Geometry check sheet. Reference: the model listing, model coordinates, mm. Round coordinates to 2 decimals unless told otherwise and drop trailing zeros. Loops run counter-clockwise (first coordinate to the right, second up) from the corner with the lowest first, then second, coordinate; pieces in that order, holes last.
```python
from build123d import *

# Parameters (mm, degrees)
SKETCH1_W                 = 3
SKETCH1_H                 = 3
PLATE_THICKNESS_3MM_DEPTH = 3
SKETCH_1_W                = 10
SKETCH_1_H                = 3
SKETCH_1_W_2              = 3
SKETCH_1_H_2              = 5
CUT_EXTRUDE_1_DEPTH       = 3


with BuildPart() as part:
    # Sketch1 → Plate_thickness_3mm (new body)
    with BuildSketch(Plane.XY):
        Polygon((30, -55), (-30, -55), (-30, -58), (-43, -58), (-43, -55), (-41.5, -55), (-41.5, -50), (-43, -50), (-43, -46), (-47, -46), (-47, -50), (-48.5, -50), (-48.5, -55), (-47, -55), (-47, -58), (-60, -58), (-60, -55), (-90, -55), (-90, 55), (-60, 55), (-60, 58), (-47, 58), (-47, 55), (-48.5, 55), (-48.5, 50), (-47, 50), (-47, 46), (-43, 46), (-43, 50), (-41.5, 50), (-41.5, 55), (-43, 55), (-43, 58), (-30, 58), (-30, 55), (30, 55), (30, 58), (43, 58), (43, 55), (41.5, 55), (41.5, 50), (43, 50), (43, 46), (47, 46), (47, 50), (48.5, 50), (48.5, 55), (47, 55), (47, 58), (60, 58), (60, 55), (90, 55), (90, -55), (60, -55), (60, -58), (47, -58), (47, -55), (48.5, -55), (48.5, -50), (47, -50), (47, -46), (43, -46), (43, -50), (41.5, -50), (41.5, -55), (43, -55), (43, -58), (30, -58), align=None)
        with Locations((-60, -10.785)):
            Rectangle(SKETCH1_W, SKETCH1_H, mode=Mode.SUBTRACT)
        with Locations((60, -10.785)):
            Rectangle(SKETCH1_W, SKETCH1_H, mode=Mode.SUBTRACT)
        with Locations((-70.785, 0)):
            Rectangle(SKETCH1_W, SKETCH1_H, mode=Mode.SUBTRACT)
        with Locations((-49.215, 0)):
            Rectangle(SKETCH1_W, SKETCH1_H, mode=Mode.SUBTRACT)
        with Locations((-60, 10.785)):
            Rectangle(SKETCH1_W, SKETCH1_H, mode=Mode.SUBTRACT)
        with Locations((49.215, 0)):
            Rectangle(SKETCH1_W, SKETCH1_H, mode=Mode.SUBTRACT)
        with Locations((70.785, 0)):
            Rectangle(SKETCH1_W, SKETCH1_H, mode=Mode.SUBTRACT)
        with Locations((60, 10.785)):
            Rectangle(SKETCH1_W, SKETCH1_H, mode=Mode.SUBTRACT)
    extrude(amount=PLATE_THICKNESS_3MM_DEPTH)

    # 草图1 → 切除-拉伸1 (cut)
    with BuildSketch(Plane.XY.offset(3)):
        with Locations((-60, -10.785)):
            Rectangle(SKETCH_1_W, SKETCH_1_H)
        with Locations((-70.785, -2.5)):
            Rectangle(SKETCH_1_W_2, SKETCH_1_H_2)
        with Locations((-70.785, 2.5)):
            Rectangle(SKETCH_1_W_2, SKETCH_1_H_2)
        with Locations((-49.215, 2.5)):
            Rectangle(SKETCH_1_W_2, SKETCH_1_H_2)
        with Locations((-49.215, -2.5)):
            Rectangle(SKETCH_1_W_2, SKETCH_1_H_2)
        with Locations((-60, 10.785)):
            Rectangle(SKETCH_1_W, SKETCH_1_H)
        with Locations((60, 10.785)):
            Rectangle(SKETCH_1_W, SKETCH_1_H)
        with Locations((49.215, 2.5)):
            Rectangle(SKETCH_1_W_2, SKETCH_1_H_2)
        with Locations((49.215, -2.5)):
            Rectangle(SKETCH_1_W_2, SKETCH_1_H_2)
        with Locations((60, -10.785)):
            Rectangle(SKETCH_1_W, SKETCH_1_H)
        with Locations((70.785, -2.5)):
            Rectangle(SKETCH_1_W_2, SKETCH_1_H_2)
        with Locations((70.785, 2.5)):
            Rectangle(SKETCH_1_W_2, SKETCH_1_H_2)
    extrude(amount=-CUT_EXTRUDE_1_DEPTH, mode=Mode.SUBTRACT)


solid = part.part
```
1) Sectioned sample at B-B, the plane z = 1.85. State how many separate pieces and enclosed holes the cut face has, then the cut area to 3 significant figures.
Report:
separate pieces: 1
enclosed holes: 8
area: 19,700 mm2
2) Scan lines: line 1 along Y through (x, z) = (-61, 1.7) (3 decimals); line 2 along X through (y, z) = (48.5, 1.85); line 3 along X through (y, z) = (-11.5, 2.5). Record each from-to range of solid material in increasing order.
Report:
line 1: y = -55 to -12.285, -9.285 to 9.285, 12.285 to 55
line 2: x = -90 to -47, -43 to 43, 47 to 90
line 3: x = -90 to -65, -55 to 55, 65 to 90
3) Sectioned sample at A-A, the plane x = -76.5. Record the cut outline in (y, z).
Report:
outline: (-55, 0) - (55, 0) - (55, 3) - (-55, 3) - close
4) Gauge pin test, flat end, axial feed: pin 1 (0.9 mm diameter, centred on y = -56, z = 1.5, fed in from -X). Record the tip position at first contact, or that the pin passes through.
Report:
pin 1: stops at x = -60
